```python
from build123d import *

# Parameters (mm, degrees)
SKETCH1_W           = 180
SKETCH1_H           = 80
SKETCH1_R           = 23.75
BOSS_EXTRUDE1_DEPTH = 3
CUT_EXTRUDE2_DEPTH  = 3
SKETCH4_R           = 1.6
CUT_EXTRUDE3_DEPTH  = 3
SKETCH7_R           = 3
SKETCH7_R_2         = 3.5
CUT_EXTRUDE4_DEPTH  = 3
FILLET1_R           = 10
FILLET2_R           = 15
FILLET3_R           = 10
SKETCH8_R           = 3
CUT_EXTRUDE6_DEPTH  = 10
SKETCH9_R           = 1.5
CUT_EXTRUDE7_DEPTH  = 10


with BuildPart() as part:
    # Sketch1 → Boss-Extrude1 (new body)
    with BuildSketch(Plane.XY):
        Rectangle(SKETCH1_W, SKETCH1_H)
        with Locations((55, 5)):
            Circle(SKETCH1_R, mode=Mode.SUBTRACT)
        with Locations((-55, 5)):
            Circle(SKETCH1_R, mode=Mode.SUBTRACT)
    extrude(amount=BOSS_EXTRUDE1_DEPTH)

    # Sketch3 → Cut-Extrude2 (cut)
    with BuildSketch(Plane.XY.offset(3)):
        Polygon((-21, -40), (-15, -34), (15, -34), (21, -40), align=None)
    extrude(amount=-CUT_EXTRUDE2_DEPTH, mode=Mode.SUBTRACT)

    # Sketch4 → Cut-Extrude3 (cut)
    with BuildSketch(Plane.XY.offset(3)):
        with Locations((-78.5, 28)):
            Circle(SKETCH4_R)
        with Locations((-31.545874822, 28)):
            Circle(SKETCH4_R)
        with Locations((-31.5, -18)):
            Circle(SKETCH4_R)
        with Locations((-78.5, -18)):
            Circle(SKETCH4_R)
        with Locations(Location((31.5, -18, 0), (0, 0, 180))):
            Circle(SKETCH4_R)
        with Locations(Location((31.545874822, 28, 0), (0, 0, 180))):
            Circle(SKETCH4_R)
        with Locations(Location((78.5, 28, 0), (0, 0, 180))):
            Circle(SKETCH4_R)
        with Locations(Location((78.5, -18, 0), (0, 0, 180))):
            Circle(SKETCH4_R)
    extrude(amount=-CUT_EXTRUDE3_DEPTH, mode=Mode.SUBTRACT)

    # Sketch7 → Cut-Extrude4 (cut)
    with BuildSketch(Plane.XY.offset(3)):
        Circle(SKETCH7_R)
        with Locations((0, 30)):
            Circle(SKETCH7_R_2)
    extrude(amount=-CUT_EXTRUDE4_DEPTH, mode=Mode.SUBTRACT)

    # Fillet1
    fillet1_edges = [part.edges().sort_by_distance(p)[0] for p in [
        (-90, 40, 1.5),
        (90, 40, 1.5),
    ]]
    fillet(fillet1_edges, radius=FILLET1_R)

    # Fillet2
    fillet2_edges = [part.edges().sort_by_distance(p)[0] for p in [
        (90, -40, 1.5),
        (-90, -40, 1.5),
    ]]
    fillet(fillet2_edges, radius=FILLET2_R)

    # Fillet3
    fillet3_edges = [part.edges().sort_by_distance(p)[0] for p in [
        (-15, -34, 1.5),
        (15, -34, 1.5),
        (21, -40, 1.5),
        (-21, -40, 1.5),
    ]]
    fillet(fillet3_edges, radius=FILLET3_R)

    # Sketch8 → Cut-Extrude6 (cut)
    with BuildSketch(Plane.XY.offset(3)):
        with Locations((-55, -29.8)):
            Circle(SKETCH8_R)
        with Locations((-73.9, -29.8)):
            Circle(SKETCH8_R)
        with Locations((55, -29.8)):
            Circle(SKETCH8_R)
        with Locations((73.9, -29.8)):
            Circle(SKETCH8_R)
        with Locations((-16.722937411, 14.75)):
            Circle(SKETCH8_R)
        with Locations((16.722937411, 14.75)):
            Circle(SKETCH8_R)
    extrude(amount=-CUT_EXTRUDE6_DEPTH, mode=Mode.SUBTRACT)

    # Sketch9 → Cut-Extrude7 (cut)
    with BuildSketch(Plane(origin=(0, 0, 0), x_dir=(-1, 0, 0), z_dir=(0, 0, -1))):
        with Locations((-21.9, -33.770050686)):
            Circle(SKETCH9_R)
        with Locations((-21.9, -13.770050686)):
            Circle(SKETCH9_R)
        with Locations(Location((21.782825633, -13.770050686, 0), (0, 0, 180))):
            Circle(SKETCH9_R)
        with Locations(Location((21.782825633, -33.770050686, 0), (0, 0, 180))):
            Circle(SKETCH9_R)
    extrude(amount=-CUT_EXTRUDE7_DEPTH, mode=Mode.SUBTRACT)


solid = part.part
```
Geometry check sheet. Reference: the model listing, model coordinates, mm. A direction names the side the tool comes from. Coordinates: 2 decimals unless noted, no trailing zeros. Order: outer loops, then holes, each group sorted by start corner. A loop starts at its lowest first (then second) coordinate and runs counter-clockwise, first axis right, second up. Notation, with made-up numbers: (-26, 9) - (13, 9) arc R23 ccw to (13, 39) - close; hole circle Ø7 at (48, -16.75). An arc over 180 degrees is marked (long way). Answer as a JSON object with one key per item and string values. Group by question number.
Item 1: Draft check along X on faces 3 (the face through (30.69, 26.65, 1.52)), 4 (the face through (-1, 40, 1)), 5 (the face through (-85.72, -35.49, 1.52)). Enter one of: +X half, -X half, draft (parallel to the pull), parting line (faces both ways), or undercut.
Item 2: Tool access check on faces 1 (the face through (-33.061, -4.096, 1.479)), 2 (the face through (14.63, -34.74, 1.48)). Record the directions out of +Z, -Z, +X, -X, +Y, -Y that give a thin tool (end or side, any length) a straight path to the whole face; none if there is none.
Item 3: Scan lines: probe 1 along Y at (x, z) = (-55, 0.7); probe 2 along X at (y, z) = (14.5, 2.8); probe 3 along Y at (x, z) = (-73.9, 1.4). Record each from-to range of solid material in increasing order.
Item 4: Sectioned sample at A-A, the plane y = 5. Record the cut outline in (x, z), and give its area (3 significant figures).
Item 5: Depth check by flat-ended pin: pin 1 Ø6 at (x, y) = (19.5, 18.5) entering from -Z. Enter the tip coordinate at first touch or a pass-through.
Item 6: Sectioned sample at B-B, the plane x = 0. Record the cut outline in (y, z).
Item 7: Sectioned sample at C-C, the plane x = -36. Record the cut outline in (y, z).
Item 8: Sectioned sample at D-D, the plane z = 1.25. Give the number of separate pieces and of enclosed holes in the cut face, and give its area (3 significant figures).
Resolved:
{
 "1": {"face 3": "undercut", "face 4": "draft", "face 5": "-X half"},
 "2": {"face 1": "+Z, -Z", "face 2": "+Z, -Z, -Y"},
 "3": {"probe 1": "-40 to -32.8, -26.8 to -18.75, 28.75 to 40", "probe 2": "-90 to -76.77, -33.23 to -19.71, -13.73 to 13.73, 19.71 to 33.23, 76.77 to 90", "probe 3": "-40 to -32.8, -26.8 to -9.38, 19.38 to 40"},
 "4": {"outline": "(-90, 0) - (-78.75, 0) - (-78.75, 3) - (-90, 3) - close; (-31.25, 0) - (31.25, 0) - (31.25, 3) - (-31.25, 3) - close; (78.75, 0) - (90, 0) - (90, 3) - (78.75, 3) - close", "area": "255 mm^2"},
 "5": {"pin 1": "z = 0"},
 "6": {"outline": "(-34, 0) - (-3, 0) - (-3, 3) - (-34, 3) - close; (3, 0) - (26.5, 0) - (26.5, 3) - (3, 3) - close; (33.5, 0) - (40, 0) - (40, 3) - (33.5, 3) - close"},
 "7": {"outline": "(-40, 0) - (-9.25, 0) - (-9.25, 3) - (-40, 3) - close; (19.25, 0) - (40, 0) - (40, 3) - (19.25, 3) - close"},
 "8": {"separate pieces": "1", "enclosed holes": "22", "area": "10,200 mm^2"}
}
